```python
from build123d import *

# Parameters (mm, degrees)
CUT_EXTRUDE1_DEPTH = 3.095625


with BuildPart() as part:
    # Sketch3 → Revolve1 (revolve)
    with BuildSketch(Plane(origin=(0, 0, 0), x_dir=(0, 0, -1), z_dir=(1, 0, 0)), mode=Mode.PRIVATE) as revolve1_sk:
        with BuildLine():
            Line((-51.59375, 0), (-51.59375, 4.28625))
            Line((-51.59375, 4.28625), (-51.1175, 4.7625))
            Line((-51.1175, 4.7625), (-47.069375, 4.7625))
            Line((-47.069375, 4.7625), (-46.83125, 4.524375))
            Line((-46.83125, 4.524375), (-46.83125, 3.1353125))
            ThreePointArc((-46.83125, 3.1353125), (-46.796377401, 3.051122599), (-46.7121875, 3.01625))
            Line((-46.7121875, 3.01625), (-45.931666667, 3.01625))
            Line((-45.931666667, 3.01625), (-45.772916667, 3.175))
            Line((-45.772916667, 3.175), (41.91, 3.175))
            Line((41.91, 3.175), (42.06875, 3.01625))
            Line((42.06875, 3.01625), (42.06875, 2.016125))
            ThreePointArc((42.06875, 2.016125), (42.184991996, 1.735491996), (42.465625, 1.61925))
            Line((42.465625, 1.61925), (43.127083333, 1.61925))
            Line((43.127083333, 1.61925), (43.920833333, 2.413))
            Line((43.920833333, 2.413), (50.8, 2.413))
            Line((50.8, 2.413), (51.59375, 1.61925))
            Line((51.59375, 1.61925), (51.59375, 0))
            Line((51.59375, 0), (-51.59375, 0))
        make_face()
    revolve(revolve1_sk.sketch.rotate(Axis((0, 0, 51.59375), (0, 0, -1)), 90), axis=Axis((0, 0, 51.59375), (0, 0, -1)))

    # Sketch4 → Cut-Extrude1 (cut)
    with BuildSketch(Plane.XY.offset(51.59375)):
        Polygon((-1.5875, -0.916543552), (0, -1.833087105), (1.5875, -0.916543552), (1.5875, 0.916543552), (0, 1.833087105), (-1.5875, 0.916543552), align=None)
    extrude(amount=-CUT_EXTRUDE1_DEPTH, mode=Mode.SUBTRACT)

    # Cut-Extrude2 cone 1 section (through the dimple's axis) → Cut-Extrude2 (revolve, cut)
    with BuildSketch(Plane(origin=(0, 0, 51.59375), x_dir=(0, -1, 0), z_dir=(1, 0, 0))):
        Polygon((0, 0), (1.833087105, 0), (0, 1.833087105), align=None)
    revolve(axis=Axis((0, 0, 51.59375), (0, 0, -1)), mode=Mode.SUBTRACT)


solid = part.part
```
For this review, take the finished solid that the model builds, in its own axes (mm). A direction names the side the tool comes from. Coordinates: 2 decimals unless noted, no trailing zeros. Write each loop counter-clockwise with the first axis right and the second up, starting at its lowest first coordinate (ties: lowest second). Pieces come first, ordered by that corner, then holes.
(1) Add section A-A on z = -20.5. Give the boundary of the cut face in (x, y) (3 decimals).
(2) Tool access review of faces 1 (the face through (2.877, -0.906, 46.316)), 2 (the face through (-1.915, 1.468, -47.409)), 3 (the face through (0, 0, -51.594)), 4 (the face through (-1.588, 0, 50)): name each direction out of +Z, -Z, +X, -X, +Y, -Y from which nothing blocks a thin tool from reaching the whole face with its end or side.
(3) Wall thickness on probe 1 along X at (y, z) = (2.75, -10.5); probe 2 along Y at (x, z) = (0, -21.5) (3 decimals); probe 3 along Z at (x, y) = (1, -3.5): over which ranges is each line inside the solid? List them lowest first.
(4) For pin 1 Ø3.5 at (x, y) = (-0.5, -1) entering from +Z; pin 2 Ø2 at (y, z) = (-0.5, -38) entering from +X (3 decimals); pin 3 Ø1.5 at (x, y) = (-3, 3.5) entering from -Z; pin 4 Ø4 at (x, z) = (-2, 19) entering from -Y (3 decimals), all flat-tipped, find the tip position at first contact; note any pin that passes through.
(5) The part is to be moulded in two halves that separate along Y. For faces 5 (the face through (-0.8, -1.37, 50.07)), 6 (the face through (-1.1, -3.1, 46.831)), 7 (the face through (-0.35, 1.58, -42.8)), 8 (the face through (0.8, 1.37, 50.07)), say which applies: +Y half, -Y half, draft (parallel to the pull), parting line (faces both ways), or undercut.
Answer sheet:
1. outline: circle Ø6.35 at (0, 0)
2. face 1: none
2. face 2: -Z
2. face 3: -Z, +X, -X, +Y, -Y
2. face 4: +Z
3. probe 1: x = -1.59 to 1.59
3. probe 2: y = -3.175 to 3.175
3. probe 3: z = 46.83 to 51.59
4. pin 1: stops at z = 51.59
4. pin 2: stops at x = 3.175
4. pin 3: stops at z = 46.83
4. pin 4: stops at y = -3.175
5. face 5: undercut
5. face 6: draft
5. face 7: parting line
5. face 8: undercut
